Autodesk Inventor part; units mm, degrees
ref_plane "YZ Plane" through (0, 0, 0) normal (1, 0, 0) x (0, 1, 0)
ref_plane "XZ Plane" through (0, 0, 0) normal (0, 1, 0) x (-1, 0, 0)
ref_plane "XY Plane" through (0, 0, 0) normal (0, 0, 1) x (1, 0, 0)
sketch "Sketch1" plane through (0, 0, 0) normal (0, 1, 0) x (-1, 0, 0)
  line L0 (-10, 75) -> (10, 75)
  line L1 (12, 73) -> (12, -75)
  line L2 (12, -75) -> (-12, -75)
  line L3 (-12, -75) -> (-12, 73)
  line L4 (-12, 75) -> (12, -75) construction
  line L5 (12, 75) -> (-12, -75) construction
  arc A0 (12, 73) -> (10, 75) centre (10, 73) ccw
  arc A1 (-10, 75) -> (-12, 73) centre (-10, 73) ccw
  circle A2 centre (8, 71) radius 2.2
  circle A3 centre (0, 71) radius 2.2
  circle A4 centre (-8, 71) radius 2.2
  circle A5 centre (8, 63) radius 2.2
  circle A6 centre (0, 63) radius 2.2
  circle A7 centre (-8, 63) radius 2.2
  point P0 (0, 0)
  dimension "d0" = 24
  dimension "d1" = 150
  dimension "d2" = 2
  dimension "d3" = 4.4
  dimension "d4" = 4
  dimension "d5" = 4
  dimension "d8" = 8
  dimension "d11" = 8
extrude "Extrusion1" add sketch "Sketch1" along normal blind 5
sketch "Sketch2" plane through (12, 0, 73) normal (1, 0, 0) x (0, 0, -1)
  arc A0 (108, 5) -> (147.1089, 23.8473) centre (108, 55) ccw
  line L0 (0, 5) -> (148, 5)
  line L1 (148, 5) -> (148, 23.5357)
  arc A1 (148, 23.5357) -> (147.1089, 23.8473) centre (147.5, 23.5357) ccw
  point P0 (73, 0)
  point P1 (148, 25)
  dimension "d16" = 100
  dimension "d17" = 40
  dimension "d18" = 0.5
extrude "Extrusion2" add sketch "Sketch2" against normal blind 24
sketch "Sketch3" plane through (12, 0, 73) normal (1, 0, 0) x (0, 0, -1)
  line L0 (0, 0) -> (148, 0)
  arc A0 (108, 5) -> (147.1089, 23.8473) centre (108, 55) ccw
  line L1 (0, 5) -> (108, 5)
  arc A1 (108, 0) -> (147.8624, 17.1055) centre (108, 55) ccw
  line L2 (148, 0) -> (148, 23.5357)
  line L3 (148, 17.2508) -> (148, 0)
  line L4 (148, 0) -> (108, 0)
  arc A2 (147.8624, 17.1055) -> (148, 17.45) centre (147.5, 17.45) ccw
  point P0 (150, 0)
  dimension "d27" = 1
  dimension "d28" = 17.2508
extrude "Extrusion3" cut sketch "Sketch3" against normal blind 24
sketch "Sketch4" plane through (12, 0, 73) normal (1, 0, 0) x (0, 0, -1)
  arc A0 (88.6931, 8.878) -> (108, 5) centre (108, 55) ccw
  line L0 (0, 5) -> (108, 5)
  line L1 (148, 17.45) -> (148, 23.5357)
  line L2 (88, 5) -> (88, 8.4167)
  arc A1 (88.6931, 8.878) -> (88, 8.4167) centre (88.5, 8.4167) ccw
  point P0 (73, 0)
  point P1 (88, 9.1742)
  dimension "d31" = 0.5
  dimension "d40" = 20
  dimension "d41" = 50
extrude "Extrusion4" add sketch "Sketch4" against normal blind 24
properties part number "Launcher_Arm_V2"
Model file for the job. Use its own axes, mm. A direction names the side the tool comes from. Coordinates: 2 decimals unless noted, no trailing zeros. Loops run counter-clockwise (first coordinate to the right, second up) from the corner with the lowest first, then second, coordinate; pieces in that order, holes last. Notation, with made-up numbers: M 23,7.25 L 75,7.25 A27 cw 75,26.25 Z; hole C 68,24.5 d9. An arc over 180 degrees is marked long. Use CSV: the item, a comma, the result in double quotes. Start each with the question number.
1. Band-saw the part on D-D, the plane z = 32. List the corners of the cut face in (x, y), then the cut area to 3 significant figures.
2. Band-saw the part on A-A, the plane z = 71. List the corners of the cut face in (x, y), then the cut area to 3 significant figures.
3. Band-saw the part on B-B, the plane x = 8. List the corners of the cut face in (y, z).
4. Probe probe 1 along Z at (x, y) = (-0.5, 4.75); probe 2 along Y at (x, z) = (7.25, 15); probe 3 along Y at (x, z) = (-1.75, -66.5). List the from-to ranges inside material, lowest first. Write a range as [from, to].
5. Two-plate mould, pull along X, no slides. Class faces 1 (the flat face through (0, 20, -75)), 2 (the cylindrical face through (-1.183, 2.465, 69.145)), 3 (the flat face through (-12, 3, -1)): pulls with the +X half, pulls with the -X half, needs draft (parallel to the pull), parting line crosses it, or undercut.
6. Flat gauge pins, fed straight in: pin 1 (4 mm diameter, centred on x = 2.5, y = 8.5, fed in from +Z); pin 2 (1 mm diameter, centred on x = -7.5, y = 4.5, fed in from -Z); pin 3 (1 mm diameter, centred on x = -9.5, y = 11, fed in from +Z). Where does each tip first touch, or does it go through?
7. Band-saw the part on C-C, the plane y = 6.5. List the corners of the cut face in (x, z).
8. Tool access for faces 4 (the cylindrical face through (0.17, 9.82, -56.42)), 5 (the flat face through (0, 0, 21)), 6 (the flat face through (0, 7, -15)): list every direction of +Z, -Z, +X, -X, +Y, -Y with a clear straight run to the whole face (end or side of a thin tool).
Entries:
1,outline,"M -12,0 L 12,0 L 12,5 L -12,5 Z"
1,area,"120 mm2"
2,outline,"M -12,0 L -10.2,0 L -10.2,5 L -12,5 Z; M -5.8,0 L -2.2,0 L -2.2,5 L -5.8,5 Z; M 2.2,0 L 5.8,0 L 5.8,5 L 2.2,5 Z; M 10.2,0 L 12,0 L 12,5 L 10.2,5 Z"
2,area,"54.0 mm2"
3,outline,"M 0,-35 A55 ccw 17.11,-74.86 A0.5 ccw 17.45,-75 L 23.54,-75 A0.5 ccw 23.85,-74.11 A50 cw 5,-35 A50 cw 8.88,-15.69 A0.5 ccw 8.42,-15 L 5,-15 L 5,60.8 L 0,60.8 Z; M 0,65.2 L 5,65.2 L 5,68.8 L 0,68.8 Z; M 0,73.2 L 5,73.2 L 5,75 L 0,75 Z"
4,probe 1,"z = [-57.36, 60.86], [65.14, 68.86], [73.14, 75]"
4,probe 2,"y = [0, 5]"
4,probe 3,"y = [9.91, 16.17]"
5,face 1,"needs draft"
5,face 2,"undercut"
5,face 3,"pulls with the -X half"
6,pin 1,"stops at z = -15"
6,pin 2,"stops at z = -57.91"
6,pin 3,"stops at z = -57.8"
7,outline,"M -12,-60.94 L 12,-60.94 L 12,-47.16 L -12,-47.16 Z; M -12,-22.84 L 12,-22.84 L 12,-15 L -12,-15 Z"
8,face 4,"+X, -X, +Y"
8,face 5,"+Z, -Z, +X, -X, -Y"
8,face 6,"+Z, +X, -X, +Y"
